```python
from build123d import *

# Parameters (mm, degrees)
BOSS_EXTRUDE1_DEPTH = 1.8
CUT_EXTRUDE1_REACH  = 3.8
SKETCH2_R           = 1.6
SKETCH3_W           = 15.875
SKETCH3_H           = 11.43
BOSS_EXTRUDE2_DEPTH = 11
SKETCH4_W           = 13.335
SKETCH4_H           = 8.89
BOSS_EXTRUDE3_DEPTH = 11
SKETCH5_W           = 20.8
SKETCH5_H           = 2.54
SKETCH5_W_2         = 5.08
SKETCH5_H_2         = 46.4
SKETCH5_W_3         = 25.4
BOSS_EXTRUDE4_DEPTH = 8.6


with BuildPart() as part:
    # Sketch1 → Boss-Extrude1 (new body)
    with BuildSketch(Plane(origin=(0, 0, 0), x_dir=(1, 0, 0), z_dir=(0, 1, 0))):
        Polygon((-49.53, -26.67), (49.53, -26.67), (49.53, -25.4), (52.07, -22.86), (52.07, 11.43), (49.53, 13.97), (49.53, 24.13), (46.99, 26.67), (-49.53, 26.67), align=None)
    extrude(amount=BOSS_EXTRUDE1_DEPTH)

    # Sketch2 → Cut-Extrude1 (cut, up to next)
    with BuildSketch(Plane(origin=(0, 1.8, 0), x_dir=(1, 0, 0), z_dir=(0, 1, 0)), mode=Mode.PRIVATE) as cut_extrude1_sk1:
        with Locations((-35.56, -24.13)):
            Circle(SKETCH2_R)
    cut_extrude1_tool1 = extrude(cut_extrude1_sk1.sketch, amount=-CUT_EXTRUDE1_REACH, mode=Mode.PRIVATE) & part.part
    add(cut_extrude1_tool1.solids().sort_by_distance((-35.56, 1.8, 24.13))[0], mode=Mode.SUBTRACT)
    # Sketch2 → Cut-Extrude1 (cut, up to next)
    with BuildSketch(Plane(origin=(0, 1.8, 0), x_dir=(1, 0, 0), z_dir=(0, 1, 0)), mode=Mode.PRIVATE) as cut_extrude1_sk2:
        with Locations((16.51, -19.05)):
            Circle(SKETCH2_R)
    cut_extrude1_tool2 = extrude(cut_extrude1_sk2.sketch, amount=-CUT_EXTRUDE1_REACH, mode=Mode.PRIVATE) & part.part
    add(cut_extrude1_tool2.solids().sort_by_distance((16.51, 1.8, 19.05))[0], mode=Mode.SUBTRACT)
    # Sketch2 → Cut-Extrude1 (cut, up to next)
    with BuildSketch(Plane(origin=(0, 1.8, 0), x_dir=(1, 0, 0), z_dir=(0, 1, 0)), mode=Mode.PRIVATE) as cut_extrude1_sk3:
        with Locations((16.51, 8.89)):
            Circle(SKETCH2_R)
    cut_extrude1_tool3 = extrude(cut_extrude1_sk3.sketch, amount=-CUT_EXTRUDE1_REACH, mode=Mode.PRIVATE) & part.part
    add(cut_extrude1_tool3.solids().sort_by_distance((16.51, 1.8, -8.89))[0], mode=Mode.SUBTRACT)
    # Sketch2 → Cut-Extrude1 (cut, up to next)
    with BuildSketch(Plane(origin=(0, 1.8, 0), x_dir=(1, 0, 0), z_dir=(0, 1, 0)), mode=Mode.PRIVATE) as cut_extrude1_sk4:
        with Locations((46.99, -24.13)):
            Circle(SKETCH2_R)
    cut_extrude1_tool4 = extrude(cut_extrude1_sk4.sketch, amount=-CUT_EXTRUDE1_REACH, mode=Mode.PRIVATE) & part.part
    add(cut_extrude1_tool4.solids().sort_by_distance((46.99, 1.8, 24.13))[0], mode=Mode.SUBTRACT)
    # Sketch2 → Cut-Extrude1 (cut, up to next)
    with BuildSketch(Plane(origin=(0, 1.8, 0), x_dir=(1, 0, 0), z_dir=(0, 1, 0)), mode=Mode.PRIVATE) as cut_extrude1_sk5:
        with Locations((40.64, 24.13)):
            Circle(SKETCH2_R)
    cut_extrude1_tool5 = extrude(cut_extrude1_sk5.sketch, amount=-CUT_EXTRUDE1_REACH, mode=Mode.PRIVATE) & part.part
    add(cut_extrude1_tool5.solids().sort_by_distance((40.64, 1.8, -24.13))[0], mode=Mode.SUBTRACT)
    # Sketch2 → Cut-Extrude1 (cut, up to next)
    with BuildSketch(Plane(origin=(0, 1.8, 0), x_dir=(1, 0, 0), z_dir=(0, 1, 0)), mode=Mode.PRIVATE) as cut_extrude1_sk6:
        with Locations((-34.29, 24.13)):
            Circle(SKETCH2_R)
    cut_extrude1_tool6 = extrude(cut_extrude1_sk6.sketch, amount=-CUT_EXTRUDE1_REACH, mode=Mode.PRIVATE) & part.part
    add(cut_extrude1_tool6.solids().sort_by_distance((-34.29, 1.8, -24.13))[0], mode=Mode.SUBTRACT)

    # Sketch3 → Boss-Extrude2 (add)
    with BuildSketch(Plane(origin=(0, 1.8, 0), x_dir=(1, 0, 0), z_dir=(0, 1, 0))):
        with Locations((-47.9425, 11.43)):
            Rectangle(SKETCH3_W, SKETCH3_H)
    extrude(amount=BOSS_EXTRUDE2_DEPTH)

    # Sketch4 → Boss-Extrude3 (add)
    with BuildSketch(Plane(origin=(0, 1.8, 0), x_dir=(1, 0, 0), z_dir=(0, 1, 0))):
        with Locations((-44.7675, -19.05)):
            Rectangle(SKETCH4_W, SKETCH4_H)
    extrude(amount=BOSS_EXTRUDE3_DEPTH)

    # Sketch5 → Boss-Extrude4 (add)
    with BuildSketch(Plane(origin=(0, 1.8, 0), x_dir=(1, 0, 0), z_dir=(0, 1, 0))):
        with Locations((-12.73, -24.13)):
            Rectangle(SKETCH5_W, SKETCH5_H)
        with Locations((10.07, -24.13)):
            Rectangle(SKETCH5_W, SKETCH5_H)
        with Locations((32.87, -24.13)):
            Rectangle(SKETCH5_W, SKETCH5_H)
        with Locations((45.72, 2.2)):
            Rectangle(SKETCH5_W_2, SKETCH5_H_2)
        with Locations((28.08, 24.13)):
            Rectangle(SKETCH5_W, SKETCH5_H)
        with Locations((5.28, 24.13)):
            Rectangle(SKETCH5_W, SKETCH5_H)
        with Locations((-18.82, 24.13)):
            Rectangle(SKETCH5_W_3, SKETCH5_H)
    extrude(amount=BOSS_EXTRUDE4_DEPTH)


solid = part.part
```
CAD build for the part. Positions are in the model's coordinates, mm. A direction names the side the tool comes from. Give positions to 0.01 mm unless a question says otherwise; leave off trailing zeros. Order: outer loops, then holes, each group sorted by start corner. A loop starts at its lowest first (then second) coordinate and runs counter-clockwise, first axis right, second up.
(1) Saw through at B-B, the plane y = 11.75. Give the cut face in (x, z) (3 decimals).
(2) Saw through at D-D, the plane z = -20. Give the cut face in (x, y), then the cut area to 3 significant figures.
(3) Mould opens along Z. For faces 4 (the flat face through (1, 1.8, 0)), 5 (the flat face through (48.28, 0.89, -25.38)), 6 (the flat face through (10, 6, 25.4)), 7 (the flat face through (-0.33, 6, 24)) say: released by +Z, released by -Z, zero draft, split by the parting line, or undercut.
(4) Flat gauge pins, fed straight in: pin 1 (4 mm diameter, centred on x = 46, z = -13.5, fed in from +Y); pin 2 (10 mm diameter, centred on x = 34.5, z = -16.5, fed in from +Y); pin 3 (1.5 mm diameter, centred on y = 8, z = -19, fed in from -X). Where does each tip first touch, or does it go through?
(5) Saw through at A-A, the plane z = -8.89. Give the cut face in (x, y) (3 decimals).
(6) Drill centre lines: L1, parallel to Z at x = 16.51, y = 1.4; L2, parallel to Z at x = 46.99, y = 1.45; L3, parallel to X at y = 1.1, z = -24.13. Where is each one in solid material? Low to high.
(7) Saw through at C-C, the plane x = 12.5. Give the cut face in (y, z).
(8) Tool access for faces 1 (the flat face through (-48, 7, -5.715)), 2 (the flat face through (10, 6, 22.86)), 3 (the flat face through (-13, 10.4, 24)): list every direction of +Z, -Z, +X, -X, +Y, -Y with a clear straight run to the whole face (end or side of a thin tool).
Results found:
1. outline: (-55.88, -17.145) - (-40.005, -17.145) - (-40.005, -5.715) - (-55.88, -5.715) - close; (-51.435, 14.605) - (-38.1, 14.605) - (-38.1, 23.495) - (-51.435, 23.495) - close
2. outline: (-49.53, 0) - (49.53, 0) - (49.53, 1.8) - (48.26, 1.8) - (48.26, 10.4) - (43.18, 10.4) - (43.18, 1.8) - (-49.53, 1.8) - close
2. area: 222 mm2
3. face 4: undercut
3. face 5: released by -Z
3. face 6: released by +Z
3. face 7: zero draft
4. pin 1: stops at y = 10.4
4. pin 2: stops at y = 1.8
4. pin 3: stops at x = 43.18
5. outline: (-55.88, 1.8) - (-49.53, 1.8) - (-49.53, 0) - (14.91, 0) - (14.91, 1.8) - (-40.005, 1.8) - (-40.005, 12.8) - (-55.88, 12.8) - close; (18.11, 0) - (52.07, 0) - (52.07, 1.8) - (48.26, 1.8) - (48.26, 10.4) - (43.18, 10.4) - (43.18, 1.8) - (18.11, 1.8) - close
6. L1: z = -26.67 to -10.49, -7.29 to 17.45, 20.65 to 26.67
6. L2: z = -26.67 to 22.53, 25.73 to 26.67
6. L3: x = -49.53 to -35.89, -32.69 to 39.04, 42.24 to 49.53
7. outline: (0, -26.67) - (1.8, -26.67) - (1.8, -25.4) - (10.4, -25.4) - (10.4, -22.86) - (1.8, -22.86) - (1.8, 22.86) - (10.4, 22.86) - (10.4, 25.4) - (1.8, 25.4) - (1.8, 26.67) - (0, 26.67) - close
8. face 1: -X, +Y
8. face 2: +X, +Y
8. face 3: +Z, -Z, +X, +Y
